Could you check a few things on this model? Use its own coordinates, in mm. Give positions to 0.01 mm unless a question says otherwise; leave off trailing zeros. Loops run counter-clockwise (first coordinate to the right, second up) from the corner with the lowest first, then second, coordinate; pieces in that order, holes last. Notation, with made-up numbers: (-35.5, 18.25) -> (4.5, 18.25) arc R16 cw to (4.5, 47.25) -> close; hole circle Ø4 at (54.25, -26). An arc over 180 degrees is marked (long way). Write item = value, one per line. Start each with the question number.
1) I want a section at C-C (y = -16.5). List the corners of the cut face in (x, z) for me.
2) I'm going to push flat-ended pins straight in: pin 1 Ø4 at (x, y) = (-3.5, -57) entering from +Z; pin 2 Ø10 at (x, z) = (-15, 22) entering from -Y; pin 3 Ø14 at (x, z) = (-26.5, 43.5) entering from -Y. Where does each tip first touch, or does it pass through?
3) I need wall thicknesses on probe 1 along Y at (x, z) = (20, 24.5); probe 2 along Y at (x, z) = (-46.5, 46); probe 3 along Z at (x, y) = (-0.5, -78.5). Which ranges of each line are inside material? Lowest first, please. Write a range as from..to.
4) I want a section at B-B (z = 30). List the corners of the cut face in (x, y) for me, and give its area (3 significant figures).
5) I want a section at A-A (x = 20). List the corners of the cut face in (y, z) for me.
from build123d import *

# Parameters (mm, degrees)
F0_W      = 127
F0_H      = 177.8
F1_DEPTH  = 12.7
F2_W      = 127
F2_H      = 165.1
F3_DEPTH  = 12.7
F4_W      = 127
F4_H      = 152.4
F5_DEPTH  = 12.7
F6_W      = 127
F6_H      = 139.7
F7_DEPTH  = 12.7
F8_W      = 127
F8_H      = 127
F9_DEPTH  = 12.7
F10_W     = 127
F10_H     = 114.3
F11_DEPTH = 12.7
F12_W     = 127
F12_H     = 101.6
F13_DEPTH = 12.7


with BuildPart() as f1:
    # F0 (on Top) → F1 (new body)
    with BuildSketch(Plane.XY):
        Rectangle(F0_W, F0_H)
    extrude(amount=F1_DEPTH)

    # F2 (on face) → F3 (join)
    with BuildSketch(Plane.XY.offset(12.7)):
        with Locations((0, 6.35)):
            Rectangle(F2_W, F2_H)
    extrude(amount=F3_DEPTH)

    # F4 (on face) → F5 (join)
    with BuildSketch(Plane.XY.offset(25.4)):
        with Locations((0, 12.7)):
            Rectangle(F4_W, F4_H)
    extrude(amount=F5_DEPTH)

    # F6 (on face) → F7 (join)
    with BuildSketch(Plane.XY.offset(38.1)):
        with Locations((0, 19.05)):
            Rectangle(F6_W, F6_H)
    extrude(amount=F7_DEPTH)

    # F8 (on face) → F9 (join)
    with BuildSketch(Plane.XY.offset(50.8)):
        with Locations((0, 25.4)):
            Rectangle(F8_W, F8_H)
    extrude(amount=F9_DEPTH)

    # F10 (on face) → F11 (join)
    with BuildSketch(Plane.XY.offset(63.5)):
        with Locations((0, 31.75)):
            Rectangle(F10_W, F10_H)
    extrude(amount=F11_DEPTH)

    # F12 (on face) → F13 (join)
    with BuildSketch(Plane.XY.offset(76.2)):
        with Locations((0, 38.1)):
            Rectangle(F12_W, F12_H)
    extrude(amount=F13_DEPTH)


solid = f1.part
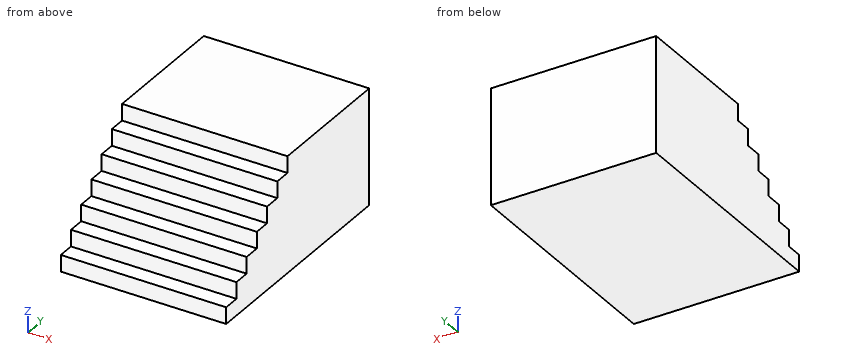
Answer list:
q1.outline = (-63.5, 0) -> (63.5, 0) -> (63.5, 76.2) -> (-63.5, 76.2) -> close
q2.pin_1 = 38.1
q2.pin_2 = -76.2
q2.pin_3 = -63.5
q3.probe_1 = -76.2..88.9
q3.probe_2 = -50.8..88.9
q3.probe_3 = 0..12.7
q4.outline = (-63.5, -63.5) -> (63.5, -63.5) -> (63.5, 88.9) -> (-63.5, 88.9) -> close
q4.area = 19,400 mm^2
q5.outline = (-88.9, 0) -> (88.9, 0) -> (88.9, 88.9) -> (-12.7, 88.9) -> (-12.7, 76.2) -> (-25.4, 76.2) -> (-25.4, 63.5) -> (-38.1, 63.5) -> (-38.1, 50.8) -> (-50.8, 50.8) -> (-50.8, 38.1) -> (-63.5, 38.1) -> (-63.5, 25.4) -> (-76.2, 25.4) -> (-76.2, 12.7) -> (-88.9, 12.7) -> close
